Drawing for the job (mm, zero at the part's lowest x, y, z). A direction names the side the tool comes from. Coordinates: 2 decimals unless noted, no trailing zeros. Order: outer loops, then holes, each group sorted by start corner. A loop starts at its lowest first (then second) coordinate and runs counter-clockwise, first axis right, second up.
1) Cut at A-A (z = 4.5). Give the number of separate pieces and of enclosed holes in the cut face.
2) Tool access for the marked faces 1 and 2: list every direction of +Z, -Z, +X, -X, +Y, -Y with a clear straight run to the whole face (end or side of a thin tool).
3) Cut at C-C (z = 16.25). List the corners of the cut face in (x, y) (1 decimal).
4) Pin check, flat tip, straight feed: pin 1 Ø7 at (x, z) = (4.5, 20.5) entering from -Y. Stop position of the tip, or through.
5) Mould opens along Z. For the marked faces 3, 4 and 5 say: +Z half, -Z half, draft (parallel to the pull), parting line (faces both ways), or undercut.
6) Cut at B-B (x = 10.5). List the corners of the cut face in (y, z) (1 decimal).
7) Wall check: L1, parallel to X at y = 1.6, z = 4.5; L2, parallel to Z at x = 12.25, y = 2.3. Give the ranges that are in metal, low to high.
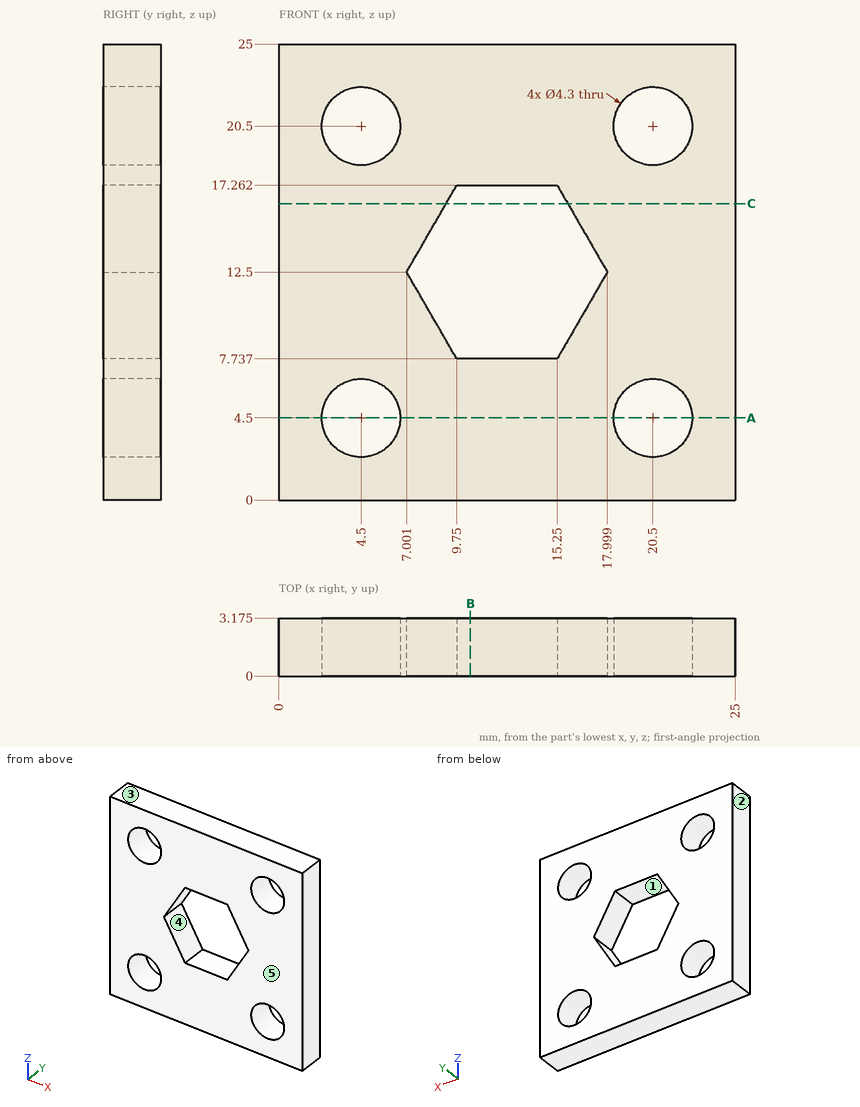
Geometry check:
1. separate pieces: 3
1. enclosed holes: 0
2. face 1: +Y, -Y
2. face 2: +Z, -Z, -X, +Y, -Y
3. outline: (0, 0) - (9.2, 0) - (9.2, 3.2) - (0, 3.2) - close; (15.8, 0) - (25, 0) - (25, 3.2) - (15.8, 3.2) - close
4. pin 1: stops at y = 0
5. face 3: +Z half
5. face 4: undercut
5. face 5: draft
6. outline: (0, 0) - (3.2, 0) - (3.2, 7.7) - (0, 7.7) - close; (0, 17.3) - (3.2, 17.3) - (3.2, 25) - (0, 25) - close
7. L1: x = 0 to 2.35, 6.65 to 18.35, 22.65 to 25
7. L2: z = 0 to 7.74, 17.26 to 25
